Input: part model. Units: mm. Frame: model coordinates. A direction names the side the tool comes from. Round coordinates to 2 decimals unless told otherwise and drop trailing zeros. Write each loop counter-clockwise with the first axis right and the second up, starting at its lowest first coordinate (ties: lowest second). Pieces come first, ordered by that corner, then holes. Notation, with made-up numbers: (87.5, 48.25) - (93.5, 48.25) arc R30 ccw to (93.5, 71.25) - close; hole circle Ø4 at (13.5, -5). An arc over 180 degrees is marked (long way). Use one line per item in the form item = value.
```python
from build123d import *

# Parameters (mm, degrees)
F0_W     = 60
F0_H     = 30
F1_DEPTH = 30
F2_W     = 30
F2_H     = 30
F3_DEPTH = 30
F3_TAPER = 10
F4_R     = 6.8568709116
F5_DEPTH = 40


with BuildPart() as f1:
    # F0 (on Front) → F1 (new body)
    with BuildSketch(Plane.XZ):
        with Locations((-1.9564672485, 1.8185370226)):
            Rectangle(F0_W, F0_H)
    extrude(amount=F1_DEPTH)

    # F2 (on face) → F3 (join)
    with BuildSketch(Plane.XY.offset(16.8185370226)):
        with Locations((13.0435327515, -15)):
            Rectangle(F2_W, F2_H)
    extrude(amount=F3_DEPTH, taper=F3_TAPER)

    # F4 (on face) → F5 (cut)
    with BuildSketch(Plane.XY.offset(46.8185370226)):
        with Locations((13.0435327515, -15)):
            Circle(F4_R)
    extrude(amount=-F5_DEPTH, mode=Mode.SUBTRACT)


solid = f1.part
```
(1) Cut plane B-B on y = -15. Output: boundary loops of the cut face in (x, z).
Derived:
outline = (-31.96, -13.18) - (28.04, -13.18) - (28.04, 16.82) - (22.75, 46.82) - (19.9, 46.82) - (19.9, 6.82) - (6.19, 6.82) - (6.19, 46.82) - (3.33, 46.82) - (-1.96, 16.82) - (-31.96, 16.82) - close
(2) Draft query along X for faces 1 (the face through (-2, -30, 2)), 2 (the face through (13, -15, 6.819)), 3 (the face through (25.436, -14.79, 31.609)), 4 (the face through (-31.956, -15, 2)). Return one class per face: released by +X, released by -X, zero draft, split by the parting line, or undercut.
Derived:
face_1 = zero draft
face_2 = undercut
face_3 = released by +X
face_4 = released by -X
(3) Access query for faces 5 (the face through (7.6, -19.17, 27.1)), 6 (the face through (12.83, -2.61, 31.61)), 7 (the face through (-17, -15, 16.819)). Directions: +Z, -Z, +X, -X, +Y, -Y. A direction counts if a zero-diameter tool reaches every point of the face in a straight line with its end or side. Return the directions, or none.
Derived:
face_5 = +Z
face_6 = +Z, +X, -X, +Y
face_7 = +Z, -X, +Y, -Y
(4) Cut plane A-A on x = 5. Output: boundary loops of the cut face in (y, z), then the cut area to 3 significant figures.
Derived:
outline = (-30, -13.18) - (0, -13.18) - (0, 16.82) - (-5.29, 46.82) - (-24.71, 46.82) - (-30, 16.82) - close
area = 1,640 mm^2
(5) Cut plane D-D on x = 19. Output: boundary loops of the cut face in (y, z), then the cut area to 3 significant figures.
Derived:
outline = (-30, -13.18) - (0, -13.18) - (0, 16.82) - (-5.29, 46.82) - (-11.6, 46.82) - (-11.6, 6.82) - (-18.4, 6.82) - (-18.4, 46.82) - (-24.71, 46.82) - (-30, 16.82) - close
area = 1,370 mm^2
(6) Material intervals for L1, parallel to Z at x = -18.5, y = -26.5; L2, parallel to Z at x = 18, y = -10.5; L3, parallel to Y at x = 10.5, z = 14.5, sorted ascending.
Derived:
L1 = -13.18 to 16.82
L2 = -13.18 to 6.82
L3 = -30 to -21.37, -8.63 to 0
(7) Cut plane C-C on z = 26.5. Output: boundary loops of the cut face in (x, y), then the cut area to 3 significant figures.
Derived:
outline = (-0.25, -28.29) - (26.34, -28.29) - (26.34, -1.71) - (-0.25, -1.71) - close; hole circle Ø13.71 at (13.04, -15)
area = 559 mm^2
(8) First-contact query: pin 1 Ø7 at (x, y) = (13, -14) entering from +Z; pin 2 Ø1.5 at (x, z) = (19.5, 22.5) entering from +Y; pin 3 Ø3 at (x, z) = (-2.5, 26.5) entering from -Y; pin 4 Ø1 at (y, z) = (-26.5, 19.5) entering from +X. Flat tips, straight axial feed; report the tip coordinate or a pass-through.
Derived:
pin_1 = 6.82
pin_2 = -0.87
pin_3 = through
pin_4 = 27.66
